Could you check a few things on this model? Use its own coordinates, in mm. Face numbers are marked on the shaded views. A direction names the side the tool comes from. Round coordinates to 2 decimals unless told otherwise and drop trailing zeros. Write each loop counter-clockwise with the first axis right and the second up, starting at its lowest first coordinate (ties: lowest second). Pieces come first, ordered by that corner, then holes. Notation, with made-up numbers: (53.25, 16) -> (64.25, 16) arc R4 ccw to (64.25, 20) -> close; hole circle Ø7 at (81, 81). An arc over 180 degrees is marked (long way). Answer in a Markdown table with one row per item. Add a question column.
```python
from build123d import *

# Parameters (mm, degrees)
SKETCH1_R           = 14.5
BOSS_EXTRUDE1_DEPTH = 120
CUT_EXTRUDE1_REACH  = 123.739
SKETCH2_R           = 12
SKETCH3_R           = 12.5
CUT_EXTRUDE2_DEPTH  = 80
CUT_EXTRUDE3_DEPTH  = 80
BOSS_EXTRUDE2_START = 2
BOSS_EXTRUDE2_DEPTH = 2
CUT_EXTRUDE4_REACH  = 125.711
CUT_EXTRUDE5_REACH  = 125.711
SKETCH7_R           = 1.25
BOSS_EXTRUDE3_DEPTH = 82
CUT_EXTRUDE6_REACH  = 124.599
SKETCH9_W           = 41
SKETCH9_H           = 6
CUT_EXTRUDE7_REACH  = 124.599
SKETCH10_R          = 2
SKETCH12_W          = 29
SKETCH12_H          = 29
BOSS_EXTRUDE4_DEPTH = 20
CUT_EXTRUDE9_REACH  = 126.557
SKETCH13_W          = 13
SKETCH13_H          = 13
CUT_EXTRUDE10_REACH = 127.145
SKETCH14_W          = 20
SKETCH14_H          = 13
CUT_EXTRUDE11_REACH = 127.145
SKETCH15_R          = 3


with BuildPart() as part:
    # Sketch1 → Boss-Extrude1 (new body)
    with BuildSketch(Plane.XY):
        Circle(SKETCH1_R)
    extrude(amount=BOSS_EXTRUDE1_DEPTH)

    # Sketch2 → Cut-Extrude1 (cut, up to next)
    with BuildSketch(Plane(origin=(0, 0, 0), x_dir=(-1, 0, 0), z_dir=(0, 0, -1)), mode=Mode.PRIVATE) as cut_extrude1_sk1:
        Circle(SKETCH2_R)
    cut_extrude1_tool1 = extrude(cut_extrude1_sk1.sketch, amount=-CUT_EXTRUDE1_REACH, mode=Mode.PRIVATE) & part.part
    add(cut_extrude1_tool1.solids().sort_by_distance((0, 0, 0))[0], mode=Mode.SUBTRACT)

    # Sketch3 → Cut-Extrude2 (cut)
    with BuildSketch(Plane(origin=(0, 0, 0), x_dir=(-1, 0, 0), z_dir=(0, 0, -1))):
        Circle(SKETCH3_R)
    extrude(amount=-CUT_EXTRUDE2_DEPTH, mode=Mode.SUBTRACT)

    # Sketch4 → Cut-Extrude3 (cut)
    with BuildSketch(Plane(origin=(0, 0, 0), x_dir=(-1, 0, 0), z_dir=(0, 0, -1))):
        with BuildLine():
            Line((0, -14.5), (0, 14.5))
            ThreePointArc((0, 14.5), (-14.5, 0), (0, -14.5))
        make_face()
    extrude(amount=-CUT_EXTRUDE3_DEPTH, mode=Mode.SUBTRACT)

    # Sketch5 → Boss-Extrude2 (add)
    with BuildSketch(Plane(origin=(0, 0, 0), x_dir=(-1, 0, 0), z_dir=(0, 0, -1)).offset(BOSS_EXTRUDE2_START)):
        with BuildLine():
            Line((0, -14.5), (0, 14.5))
            ThreePointArc((0, 14.5), (14.5, 0), (0, -14.5))
        make_face()
    extrude(amount=-BOSS_EXTRUDE2_DEPTH)

    # Sketch6 → Cut-Extrude4 (cut, up to next)
    with BuildSketch(Plane(origin=(0, 0, -2), x_dir=(-1, 0, 0), z_dir=(0, 0, -1)), mode=Mode.PRIVATE) as cut_extrude4_sk1:
        with BuildLine():
            Line((0, -3.5), (0, 3.5))
            ThreePointArc((0, 3.5), (3.5, 0), (0, -3.5))
        make_face()
    cut_extrude4_tool1 = extrude(cut_extrude4_sk1.sketch, amount=-CUT_EXTRUDE4_REACH, mode=Mode.PRIVATE) & part.part
    add(cut_extrude4_tool1.solids().sort_by_distance((-1.485446, 0, -2))[0], mode=Mode.SUBTRACT)

    # Sketch7 → Cut-Extrude5 (cut, up to next)
    with BuildSketch(Plane(origin=(0, 0, -2), x_dir=(-1, 0, 0), z_dir=(0, 0, -1)), mode=Mode.PRIVATE) as cut_extrude5_sk1:
        with Locations((8.5, 0)):
            Circle(SKETCH7_R)
    cut_extrude5_tool1 = extrude(cut_extrude5_sk1.sketch, amount=-CUT_EXTRUDE5_REACH, mode=Mode.PRIVATE) & part.part
    add(cut_extrude5_tool1.solids().sort_by_distance((-8.5, 0, -2))[0], mode=Mode.SUBTRACT)

    # Sketch8 → Boss-Extrude3 (add)
    with BuildSketch(Plane(origin=(0, 0, -2), x_dir=(-1, 0, 0), z_dir=(0, 0, -1))):
        with BuildLine():
            Line((0, -14.5), (0, -20.5))
            Line((0, -20.5), (2, -20.5))
            Line((2, -20.5), (2, -14.361406616))
            ThreePointArc((2, -14.361406616), (1.00239814, -14.465310158), (0, -14.5))
        make_face()
    boss_extrude3 = extrude(amount=-BOSS_EXTRUDE3_DEPTH)

    # Sketch9 → Cut-Extrude6 (cut, up to next)
    with BuildSketch(Plane(origin=(0, 0, 0), x_dir=(0, 0, -1), z_dir=(1, 0, 0)), mode=Mode.PRIVATE) as cut_extrude6_sk1:
        with Locations((-18.5, -17.5)):
            Rectangle(SKETCH9_W, SKETCH9_H)
    cut_extrude6_tool1 = extrude(cut_extrude6_sk1.sketch, amount=-CUT_EXTRUDE6_REACH, mode=Mode.PRIVATE) & part.part
    cut_extrude6 = cut_extrude6_tool1.solids().sort_by_distance((0, -17.5, 18.5))[0]
    add(cut_extrude6, mode=Mode.SUBTRACT)

    # Sketch10 → Cut-Extrude7 (cut, up to next)
    with BuildSketch(Plane(origin=(0, 0, 0), x_dir=(0, 0, -1), z_dir=(1, 0, 0)), mode=Mode.PRIVATE) as cut_extrude7_sk1:
        with Locations((-77, -17.5)):
            Circle(SKETCH10_R)
    cut_extrude7_tool1 = extrude(cut_extrude7_sk1.sketch, amount=-CUT_EXTRUDE7_REACH, mode=Mode.PRIVATE) & part.part
    # Sketch10 → Cut-Extrude7 (cut, up to next)
    with BuildSketch(Plane(origin=(0, 0, 0), x_dir=(0, 0, -1), z_dir=(1, 0, 0)), mode=Mode.PRIVATE) as cut_extrude7_sk2:
        with Locations((-59.5, -17.5)):
            Circle(SKETCH10_R)
    cut_extrude7_tool2 = extrude(cut_extrude7_sk2.sketch, amount=-CUT_EXTRUDE7_REACH, mode=Mode.PRIVATE) & part.part
    # Sketch10 → Cut-Extrude7 (cut, up to next)
    with BuildSketch(Plane(origin=(0, 0, 0), x_dir=(0, 0, -1), z_dir=(1, 0, 0)), mode=Mode.PRIVATE) as cut_extrude7_sk3:
        with Locations((-43, -17.5)):
            Circle(SKETCH10_R)
    cut_extrude7_tool3 = extrude(cut_extrude7_sk3.sketch, amount=-CUT_EXTRUDE7_REACH, mode=Mode.PRIVATE) & part.part
    cut_extrude7_1 = cut_extrude7_tool1.solids().sort_by_distance((0, -17.5, 77))[0]
    add(cut_extrude7_1, mode=Mode.SUBTRACT)
    cut_extrude7_2 = cut_extrude7_tool2.solids().sort_by_distance((0, -17.5, 59.5))[0]
    add(cut_extrude7_2, mode=Mode.SUBTRACT)
    cut_extrude7_3 = cut_extrude7_tool3.solids().sort_by_distance((0, -17.5, 43))[0]
    add(cut_extrude7_3, mode=Mode.SUBTRACT)
    cut_extrude7 = cut_extrude7_1 + cut_extrude7_2 + cut_extrude7_3  # Cut-Extrude7 as one shape, for the pattern or mirror that repeats it

    # Mirror1: Boss-Extrude3, Cut-Extrude6, Cut-Extrude7 across plane
    add(boss_extrude3.mirror(Plane.ZX))
    add(cut_extrude6.mirror(Plane.ZX), mode=Mode.SUBTRACT)
    add(cut_extrude7.mirror(Plane.ZX), mode=Mode.SUBTRACT)

    # Sketch12 → Boss-Extrude4 (add)
    with BuildSketch(Plane.XY.offset(120)):
        Rectangle(SKETCH12_W, SKETCH12_H)
    extrude(amount=-BOSS_EXTRUDE4_DEPTH)

    # Sketch13 → Cut-Extrude9 (cut, up to next)
    with BuildSketch(Plane.XY.offset(120), mode=Mode.PRIVATE) as cut_extrude9_sk1:
        Rectangle(SKETCH13_W, SKETCH13_H)
    cut_extrude9_tool1 = extrude(cut_extrude9_sk1.sketch, amount=-CUT_EXTRUDE9_REACH, mode=Mode.PRIVATE) & part.part
    add(cut_extrude9_tool1.solids().sort_by_distance((0, 0, 120))[0], mode=Mode.SUBTRACT)

    # Sketch14 → Cut-Extrude10 (cut, up to next)
    with BuildSketch(Plane.ZY.offset(14.5), mode=Mode.PRIVATE) as cut_extrude10_sk1:
        with Locations((110, 0)):
            Rectangle(SKETCH14_W, SKETCH14_H)
    cut_extrude10_tool1 = extrude(cut_extrude10_sk1.sketch, amount=-CUT_EXTRUDE10_REACH, mode=Mode.PRIVATE) & part.part
    add(cut_extrude10_tool1.solids().sort_by_distance((-14.5, 0, 110))[0], mode=Mode.SUBTRACT)

    # Sketch15 → Cut-Extrude11 (cut, up to next)
    with BuildSketch(Plane(origin=(14.5, 0, 0), x_dir=(0, 0, -1), z_dir=(1, 0, 0)), mode=Mode.PRIVATE) as cut_extrude11_sk1:
        with Locations(Location((-110, 0, 0), (0, 0, 90))):
            Circle(SKETCH15_R)
    cut_extrude11_tool1 = extrude(cut_extrude11_sk1.sketch, amount=-CUT_EXTRUDE11_REACH, mode=Mode.PRIVATE) & part.part
    add(cut_extrude11_tool1.solids().sort_by_distance((14.5, 0, 110))[0], mode=Mode.SUBTRACT)


solid = part.part
```
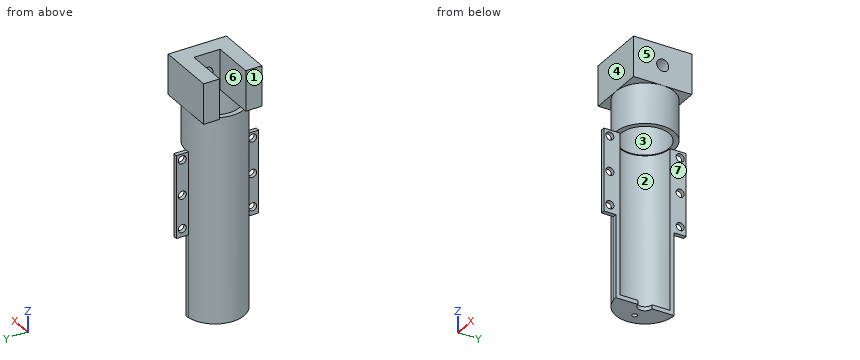
(1) I need wall thicknesses on L1, parallel to Y at x = -0.5, z = 59.5; L2, parallel to Z at x = -1.15, y = 17.5; L3, parallel to Y at x = -1.55, z = 59.5. Which ranges of each line are inside material? Lowest first, please.
(2) If we mould it in two halves opening along X, with no side actions, what happens to the marked faces 1, 2, 3 and 4? For each: pulls with the +X half, pulls with the -X half, needs draft (parallel to the pull), parting line crosses it, or undercut.
(3) For P1, Ø1, axis at y = -1, z = 67.5, coming from the -X side; P2, Ø5, axis at y = -17.5, z = 77, coming from the +X side; P3, Ø2.5, axis at y = 17.5, z = 77, coming from the -X side; P4, Ø10, axis at x = -7.5, z = 109, coming from the -Y side, each with a flat end and sliding along its axis, tell me the tip position at first contact or that it passes through.
(4) Suppose I cut it at D-D, the plane z = 43. Please give me the cut outline in (x, y).
(5) Suppose I cut it at C-C, the plane x = 4. Please give me the cut outline in (y, z).
(6) Suppose I cut it at A-A, the plane y = 17.5. Please give me the cut outline in (x, z), then the cut area to 3 significant figures.
(7) Suppose I cut it at B-B, the plane z = 110. Please give me the cut outline in (x, y), then the cut area to 3 significant figures.
(8) On a 3-axis mill with a long thin cutter (end or side, diameter ignored), from which of +Z, -Z, +X, -X, +Y, -Y can I reach the whole of each face in a straight line? I mean the marked faces 5, 6 and 7. Say none if no direction works.
Response:
| question | item | result |
|---|---|---|
| 1 | L1 | -20.5 to -19.5, -15.5 to -12.49, 12.49 to 15.5, 19.5 to 20.5 |
| 1 | L2 | 39 to 41, 45 to 57.5, 61.5 to 75, 79 to 80 |
| 1 | L3 | -20.5 to -19.5, -15.5 to -12.4, 12.4 to 15.5, 19.5 to 20.5 |
| 2 | face 1 | pulls with the -X half |
| 2 | face 2 | pulls with the +X half |
| 2 | face 3 | undercut |
| 2 | face 4 | needs draft |
| 3 | P1 | x = -14.49 |
| 3 | P2 | x = 0 |
| 3 | P3 | through |
| 3 | P4 | y = -14.5 |
| 4 | outline | (-2, -20.5) -> (0, -20.5) -> (0, -19.5) -> (-2, -19.5) -> close; (-2, -15.5) -> (0, -15.5) -> (0, -12.5) arc R12.5 cw to (0, 12.5) -> (0, 15.5) -> (-2, 15.5) -> (-2, 14.36) arc R14.5 ccw to (-2, -14.36) -> close; (-2, 19.5) -> (0, 19.5) -> (0, 20.5) -> (-2, 20.5) -> close |
| 5 | outline | (-14.5, 100) -> (-13.94, 100) -> (-13.94, 80) -> (-11.31, 80) -> (-11.31, 100) -> (-6.5, 100) -> (-6.5, 120) -> (-14.5, 120) -> close; (6.5, 100) -> (11.31, 100) -> (11.31, 80) -> (13.94, 80) -> (13.94, 100) -> (14.5, 100) -> (14.5, 120) -> (6.5, 120) -> close |
| 6 | outline | (-2, 39) -> (0, 39) -> (0, 41) -> (-2, 41) -> close; (-2, 45) -> (0, 45) -> (0, 57.5) -> (-2, 57.5) -> close; (-2, 61.5) -> (0, 61.5) -> (0, 75) -> (-2, 75) -> close; (-2, 79) -> (0, 79) -> (0, 80) -> (-2, 80) -> close |
| 6 | area | 58.0 mm² |
| 7 | outline | (-14.5, -14.5) -> (14.5, -14.5) -> (14.5, -3) -> (6.5, -3) -> (6.5, -6.5) -> (-14.5, -6.5) -> close; (-14.5, 6.5) -> (6.5, 6.5) -> (6.5, 3) -> (14.5, 3) -> (14.5, 14.5) -> (-14.5, 14.5) -> close |
| 7 | area | 520 mm² |
| 8 | face 5 | +Z, -Z, +X, +Y, -Y |
| 8 | face 6 | +Z, -X |
| 8 | face 7 | -Z, +X, +Y, -Y |
